Read the model definition and answer for the solid it produces. Units are mm, in the model's axes. Face numbers are marked on the shaded views. A direction names the side the tool comes from. Coordinates: 2 decimals unless noted, no trailing zeros. Write each loop counter-clockwise with the first axis right and the second up, starting at its lowest first coordinate (ties: lowest second). Pieces come first, ordered by that corner, then holes. Notation, with made-up numbers: (-37.75, 26.5) -> (-33.75, 26.5) arc R15 ccw to (-33.75, 32.5) -> close; hole circle Ø5 at (51, 7.25). An arc over 180 degrees is marked (long way). One line per item, written item: value. Start each with the question number.
1. Given P1, Ø8.5, axis at x = 15, z = -34, coming from the +Y side; P2, Ø1.5, axis at x = 9.5, y = 41.5, coming from the +Z side; P3, Ø18.5, axis at y = 34.5, z = 1, coming from the +X side, each flat-ended and moving along its own axis, determine where each tip first touches the part or whether it passes through.
2. Find section B-B, the plane z = -2.5. Write down the section's boundary in (x, y), and give its area (3 significant figures).
3. Find section D-D, the plane y = 32. Write down the section's boundary in (x, z), and give its area (3 significant figures).
4. Find section C-C, the plane y = 76.5. Write down the section's boundary in (x, z).
5. Consider line 1 along X through (y, z) = (81, -34); line 2 along Z through (x, y) = (7, 19); line 3 along Y through (x, z) = (7.75, -5). Determine where each line is inside the solid, lowest interval first.
6. Find section A-A, the plane x = 15. Write down the section's boundary in (y, z).
7. For a pull along Z with two mould halves and no side action, classify the marked faces 1, 2 and 3 as pulls with the +Z half, pulls with the -Z half, needs draft (parallel to the pull), parting line crosses it, or undercut.
8. For the marked faces 4, 5, 6 and 7, determine the directions among +Z, -Z, +X, -X, +Y, -Y from which every point of the face is accessible in a straight line to the end or side of a thin tool.
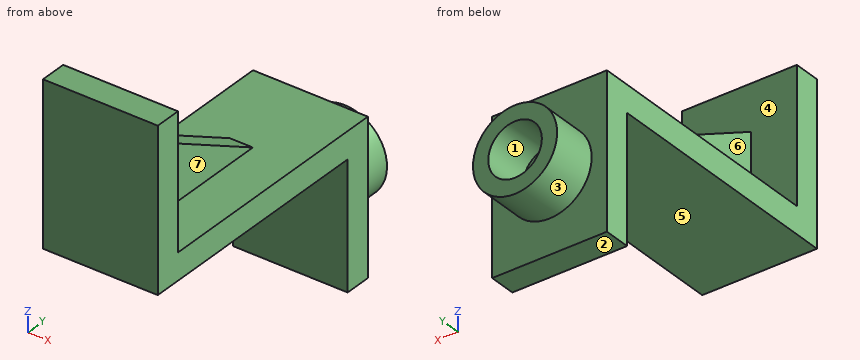
```python
from build123d import *

# Parameters (mm, degrees)
SKETCH1_W           = 30
SKETCH1_H           = 66
BOSS_EXTRUDE1_DEPTH = 21
SKETCH2_W           = 30
SKETCH2_H           = 59
CUT_EXTRUDE1_DEPTH  = 84.785440263
SKETCH4_W           = 30
SKETCH4_H           = 7
BOSS_EXTRUDE2_DEPTH = 66
SKETCH9_W           = 30
SKETCH9_H           = 7
BOSS_EXTRUDE3_DEPTH = 40
SKETCH10_R          = 11
SKETCH10_R_2        = 7
BOSS_EXTRUDE4_DEPTH = 12
BOSS_EXTRUDE6_DEPTH = 3


with BuildPart() as part:
    # Sketch1 → Boss-Extrude1 (new, symmetric)
    with BuildSketch(Plane.XY):
        with Locations((15, 33)):
            Rectangle(SKETCH1_W, SKETCH1_H)
    extrude(amount=BOSS_EXTRUDE1_DEPTH, both=True)

    # Sketch2 → Cut-Extrude1 (cut, through all)
    with BuildSketch(Plane.XY.offset(21)):
        with Locations((15, 36.5)):
            Rectangle(SKETCH2_W, SKETCH2_H)
    extrude(amount=-CUT_EXTRUDE1_DEPTH, mode=Mode.SUBTRACT)

    # Sketch4 → Boss-Extrude2 (add)
    with BuildSketch(Plane(origin=(0, 7, 0), x_dir=(1, 0, 0), z_dir=(0, 1, 0))):
        with Locations((15, 17.5)):
            Rectangle(SKETCH4_W, SKETCH4_H)
    extrude(amount=BOSS_EXTRUDE2_DEPTH)

    # Sketch9 → Boss-Extrude3 (add)
    with BuildSketch(Plane.XY.offset(-14)):
        with Locations((15, 69.5)):
            Rectangle(SKETCH9_W, SKETCH9_H)
    extrude(amount=-BOSS_EXTRUDE3_DEPTH)

    # Sketch10 → Boss-Extrude4 (add)
    with BuildSketch(Plane(origin=(0, 73, 0), x_dir=(1, 0, 0), z_dir=(0, 1, 0))):
        with Locations(Location((15, 34, 0), (0, 0, 90))):
            Circle(SKETCH10_R)
        with Locations(Location((15, 34, 0), (0, 0, 270))):
            Circle(SKETCH10_R_2, mode=Mode.SUBTRACT)
    extrude(amount=BOSS_EXTRUDE4_DEPTH)

    # Sketch18 → Boss-Extrude6 (add, symmetric)
    with BuildSketch(Plane(origin=(15, 0, 0), x_dir=(0, 0, -1), z_dir=(1, 0, 0))):
        Polygon((14, 49), (-9, 7), (14, 7), align=None)
    extrude(amount=BOSS_EXTRUDE6_DEPTH, both=True)


solid = part.part
```
Answer block:
1. P1: stops at y = 73
1. P2: stops at z = -14
1. P3: stops at x = 18
2. outline: (0, 0) -> (30, 0) -> (30, 7) -> (18, 7) -> (18, 28) -> (12, 28) -> (12, 7) -> (0, 7) -> close
2. area: 336 mm2
3. outline: (0, -21) -> (30, -21) -> (30, -14) -> (18, -14) -> (18, -4.69) -> (12, -4.69) -> (12, -14) -> (0, -14) -> close
3. area: 266 mm2
4. outline: circle Ø22 at (15, -34); hole circle Ø14 at (15, -34)
5. line 1: x = 4 to 8, 22 to 26
5. line 2: z = -21 to -14
5. line 3: y = 0 to 7
6. outline: (0, -21) -> (66, -21) -> (66, -54) -> (73, -54) -> (73, -45) -> (85, -45) -> (85, -41) -> (73, -41) -> (73, -27) -> (85, -27) -> (85, -23) -> (73, -23) -> (73, -14) -> (49, -14) -> (7, 9) -> (7, 21) -> (0, 21) -> close
7. face 1: undercut
7. face 2: pulls with the -Z half
7. face 3: parting line crosses it
8. face 4: +Z, +Y
8. face 5: -Z, +X, -X, -Y
8. face 6: +Z, -X, +Y
8. face 7: +Z, +X, +Y
